from build123d import *

# Parameters (mm, degrees)
BOSS_EXTRUDE1_START = -0.0001
SKETCH2_W           = 100
SKETCH2_H           = 30
BOSS_EXTRUDE1_DEPTH = 5.0001
CIRPATTERN1_COUNT   = 2
CIRPATTERN1_ANGLE   = 60
SKETCH4_R           = 3
CUT_EXTRUDE1_DEPTH  = 10
SKETCH5_R           = 3
CUT_EXTRUDE2_DEPTH  = 10


with BuildPart() as part:
    # Sketch2 → Boss-Extrude1 (new body)
    with BuildSketch(Plane(origin=(0, 0, 0), x_dir=(1, 0, 0), z_dir=(0, 1, 0)).offset(BOSS_EXTRUDE1_START)):
        Rectangle(SKETCH2_W, SKETCH2_H)
    boss_extrude1 = extrude(amount=BOSS_EXTRUDE1_DEPTH)

    # CirPattern1: Boss-Extrude1 ×2 about axis
    cirpattern1_axis = Axis((0, -0.0001, 15), (-1, 0, 0))
    for i in range(1, CIRPATTERN1_COUNT):
        add(boss_extrude1.rotate(cirpattern1_axis, i * CIRPATTERN1_ANGLE / (CIRPATTERN1_COUNT - 1)))

    # Sketch4 → Cut-Extrude1 (cut)
    with BuildSketch(Plane.XZ.offset(0.0001)):
        Circle(SKETCH4_R)
        with Locations((40, 0)):
            Circle(SKETCH4_R)
        with Locations((-40, 0)):
            Circle(SKETCH4_R)
    extrude(amount=-CUT_EXTRUDE1_DEPTH, mode=Mode.SUBTRACT)

    # Sketch5 → Cut-Extrude2 (cut)
    with BuildSketch(Plane(origin=(0, -6.495215528, 11.250043301), x_dir=(1, 0, 0), z_dir=(0, -0.5, 0.866025404))):
        with Locations((40, -4.500086603)):
            Circle(SKETCH5_R)
        with Locations((0, -4.500086603)):
            Circle(SKETCH5_R)
        with Locations((-40, -4.500086603)):
            Circle(SKETCH5_R)
    extrude(amount=-CUT_EXTRUDE2_DEPTH, mode=Mode.SUBTRACT)


solid = part.part
Geometry check sheet. Reference: the model listing, model coordinates, mm. A direction names the side the tool comes from. Give positions to 0.01 mm unless a question says otherwise; leave off trailing zeros. Write each loop counter-clockwise with the first axis right and the second up, starting at its lowest first coordinate (ties: lowest second). Pieces come first, ordered by that corner, then holes. Notation, with made-up numbers: M -15,41 L 34,41 A18 ccw 34,47 Z; hole C 38,40 d3. An arc over 180 degrees is marked long. One line per question, with ' | ' between items.
1. Cross-section at C-C (x = -39.5). Enter the section's corners in (y, z), plus the area to 3 significant figures.
Ans:
outline: M -25.98,0 L -23.48,-4.33 L -10.45,3.19 L -12.95,7.52 Z; M -7.83,10.48 L -5.33,6.15 L 0,9.23 L 0,2.96 L 5,2.96 L 5,15 L 0,15 Z; M 0,-15 L 5,-15 L 5,-2.96 L 0,-2.96 Z | area: 234 mm2
2. Mould release check, pull along Y, two halves, no side actions. Record for faces 4 (the face through (-3, 2, 0)), 5 (the face through (-0.7, -24.75, -2.13)), 6 (the face through (-0.7, -11.905, 2.353)): released by +Y, released by -Y, zero draft, split by the parting line, or undercut.
Ans:
face 4: zero draft | face 5: released by -Y | face 6: undercut
3. Cross-section at D-D (x = 40). Enter the section's corners in (y, z), plus the area to 3 significant figures.
Ans:
outline: M -25.98,0 L -23.48,-4.33 L -10.49,3.17 L -12.99,7.5 Z; M -7.79,10.5 L -5.29,6.17 L 0,9.23 L 0,3 L 5,3 L 5,15 L 0,15 Z; M 0,-15 L 5,-15 L 5,-3 L 0,-3 Z | area: 233 mm2
4. Scan lines: line 1 along Z through (x, y) = (40, 2); line 2 along Y through (x, z) = (34, -0.25); line 3 along Y through (x, z) = (18.5, 8). Record each from-to range of solid material in increasing order. Write a range as from..to.
Ans:
line 1: -15..-3, 3..15 | line 2: -25.84..-16.41, 0..5 | line 3: -12.12..-2.12, 0..5
5. Cross-section at A-A (x = 19). Enter the section's corners in (y, z), plus the area to 3 significant figures.
Ans:
outline: M -25.98,0 L -23.48,-4.33 L 0,9.23 L 0,-15 L 5,-15 L 5,15 L 0,15 Z | area: 293 mm2
6. Cross-section at B-B (z = 1.5). Enter the section's corners in (x, y), plus the area to 3 significant figures.
Ans:
outline: M -50,-23.38 L 50,-23.38 L 50,-13.38 L -50,-13.38 Z; M -50,0 L -42.6,0 L -42.6,5 L -50,5 Z; M -37.4,0 L -2.6,0 L -2.6,5 L -37.4,5 Z; M 2.6,0 L 37.4,0 L 37.4,5 L 2.6,5 Z; M 42.6,0 L 50,0 L 50,5 L 42.6,5 Z | area: 1,420 mm2
7. Gauge pin test, flat ends, axial feed: pin 1 (2 mm diameter, centred on x = -4.5, z = 5.5, fed in from -Y); pin 2 (6 mm diameter, centred on x = -2.5, z = -6, fed in from -Y); pin 3 (6 mm diameter, centred on x = -17.5, y = -19.5, fed in from +Z). Record the tip position at first contact, or that the pin passes through.
Ans:
pin 1: y = -18.19 | pin 2: y = -24.25 | pin 3: z = 5.47
8. Set-up check for faces 1 (the face through (37, 2, 0)), 2 (the face through (-1, 0, -3)), 3 (the face through (-1, 2, -15)): record each of +Z, -Z, +X, -X, +Y, -Y from which the full face is reachable in a straight line by a thin tool's end or side.
Ans:
face 1: +Y | face 2: -Z, +X, -X | face 3: -Z, +X, -X, +Y, -Y
